```python
from build123d import *

# Parameters (mm, degrees)
SKETCH1_W                   = 57.6
SKETCH1_H                   = 31.2
BOSS_EXTRUDE1_DEPTH         = 15
FILLET1_R                   = 7.5
SHELL1_START                = -27.8
SHELL1_DEPTH                = 55.6
SKETCH4_W                   = 2.5
SKETCH4_H                   = 7.5
SKETCH4_W_2                 = 20.6
CUT_EXTRUDE1_DEPTH          = 46.03198863
SKETCH5_R                   = 1.4
CUT_EXTRUDE2_DEPTH          = 15
M3_TAPPED_HOLE1_D           = 2.5
M3_TAPPED_HOLE1_DEPTH       = 16
M3_TAPPED_HOLE1_CSINK_D     = 6
M3_TAPPED_HOLE1_CSINK_ANGLE = 90
M3_TAPPED_HOLE1_TIP         = 0.751075774


# Read off the part's stored shape, not the designer's step: Shell1
with BuildPart() as part:
    # Sketch1 → Boss-Extrude1 (new body)
    with BuildSketch(Plane(origin=(0, 0, 0), x_dir=(1, 0, 0), z_dir=(0, 1, 0))):
        Rectangle(SKETCH1_W, SKETCH1_H)
    extrude(amount=BOSS_EXTRUDE1_DEPTH)

    # Fillet1
    fillet1_edges = [part.edges().sort_by_distance(p)[0] for p in [
        (0, 15, 15.6),
        (0, 15, -15.6),
    ]]
    fillet(fillet1_edges, radius=FILLET1_R)

    # Shell1 outline → Shell1 (cut)
    with BuildSketch(Plane.YZ.offset(SHELL1_START)):
        with BuildLine():
            Line((15, -8.1), (15, 8.1))
            Line((15, 8.1), (14, 8.1))
            ThreePointArc((14, 8.1), (12.096194078, 12.696194078), (7.5, 14.6))
            Line((7.5, 14.6), (1, 14.6))
            Line((1, 14.6), (1, -14.6))
            Line((1, -14.6), (7.5, -14.6))
            ThreePointArc((7.5, -14.6), (12.096194078, -12.696194078), (14, -8.1))
            Line((14, -8.1), (15, -8.1))
        make_face()
    extrude(amount=SHELL1_DEPTH, mode=Mode.SUBTRACT)

    # Sketch4 → Cut-Extrude1 (cut, through all)
    with BuildSketch(Plane.XY.offset(15.6)):
        with Locations((-26.55, 11.25)):
            Rectangle(SKETCH4_W, SKETCH4_H)
        with Locations((0, 11.25)):
            Rectangle(SKETCH4_W_2, SKETCH4_H)
        with Locations((26.55, 11.25)):
            Rectangle(SKETCH4_W, SKETCH4_H)
    extrude(amount=-CUT_EXTRUDE1_DEPTH, mode=Mode.SUBTRACT)

    # Sketch5 → Cut-Extrude2 (cut)
    with BuildSketch(Plane(origin=(0, 1, 0), x_dir=(1, 0, 0), z_dir=(0, 1, 0))):
        with Locations(Location((0, 0, 0), (0, 0, 270))):
            Circle(SKETCH5_R)
        with Locations(Location((7.2, 0, 0), (0, 0, 270))):
            Circle(SKETCH5_R)
        with Locations(Location((-7.2, 0, 0), (0, 0, 270))):
            Circle(SKETCH5_R)
    extrude(amount=-CUT_EXTRUDE2_DEPTH, mode=Mode.SUBTRACT)

    # M3 Tapped Hole1
    with Locations(Plane(origin=(0, 1, 31.4), x_dir=(1, 0, 0), z_dir=(0, 1, 0))):
        with Locations((7.2, 31.4), (0, 31.4), (-7.2, 31.4)):
            CounterSinkHole(M3_TAPPED_HOLE1_D / 2, M3_TAPPED_HOLE1_CSINK_D / 2, depth=M3_TAPPED_HOLE1_DEPTH, counter_sink_angle=M3_TAPPED_HOLE1_CSINK_ANGLE)
            with Locations((0, 0, -(M3_TAPPED_HOLE1_DEPTH + M3_TAPPED_HOLE1_TIP / 2))):  # 118° drill point
                Cone(0, M3_TAPPED_HOLE1_D / 2, M3_TAPPED_HOLE1_TIP, mode=Mode.SUBTRACT)


solid = part.part
```
Check sheet for the modelled part. Datum: model origin and axes. Units: mm. A direction names the side the tool comes from. Give positions to 0.01 mm unless a question says otherwise; leave off trailing zeros. Order: outer loops, then holes, each group sorted by start corner. A loop starts at its lowest first (then second) coordinate and runs counter-clockwise, first axis right, second up. Notation, with made-up numbers: (44.25, -36) -> (97.25, -36) arc R31 ccw to (97.25, -7) -> close; hole circle Ø10 at (44, 30). An arc over 180 degrees is marked (long way). Return JSON: item names as keys, results as strings.
1. Material ranges on probe 1 along Z at (x, y) = (-3, 2.5); probe 2 along X at (y, z) = (9.75, 11); probe 3 along Y at (x, z) = (-14.5, -7), recorded low to high. Write a range as [from, to].
From the geometry:
{"probe 1": "[-15.6, -14.6], [14.6, 15.6]", "probe 2": "[-28.8, -27.8], [27.8, 28.8]", "probe 3": "[0, 1]"}
2. Mould release check, pull along Y, two halves, no side actions. Record for faces 4 (the cylindrical face through (-28.293, 12.745, -13.461)), 5 (the cylindrical face through (17.695, 12.045, -12.746)), 6 (the flat face through (-25.3, 12, 13)): +Y half, -Y half, draft (parallel to the pull), parting line (faces both ways), or undercut.
From the geometry:
{"face 4": "+Y half", "face 5": "undercut", "face 6": "draft"}
3. Cross-section at A-A, the plane x = -7.2. Record the cut outline in (y, z), plus the area to 3 significant figures.
From the geometry:
{"outline": "(0, -15.6) -> (7.5, -15.6) -> (7.5, -14.6) -> (1, -14.6) -> (1, -3) -> (0, -2) -> close; (0, 2) -> (1, 3) -> (1, 14.6) -> (7.5, 14.6) -> (7.5, 15.6) -> (0, 15.6) -> close", "area": "39.2 mm^2"}
4. Cross-section at D-D, the plane y = 11.75. Record the cut outline in (x, z), plus the area to 3 significant figures.
From the geometry:
{"outline": "(-28.8, -14.28) -> (-27.8, -14.28) -> (-27.8, 14.28) -> (-28.8, 14.28) -> close; (-25.3, -14.28) -> (-10.3, -14.28) -> (-10.3, -13.02) -> (-25.3, -13.02) -> close; (-25.3, 13.02) -> (-10.3, 13.02) -> (-10.3, 14.28) -> (-25.3, 14.28) -> close; (10.3, -14.28) -> (25.3, -14.28) -> (25.3, -13.02) -> (10.3, -13.02) -> close; (10.3, 13.02) -> (25.3, 13.02) -> (25.3, 14.28) -> (10.3, 14.28) -> close; (27.8, -14.28) -> (28.8, -14.28) -> (28.8, 14.28) -> (27.8, 14.28) -> close", "area": "133 mm^2"}
5. Set-up check for faces 1 (the flat face through (0, 4, -14.6)), 2 (the cylindrical face through (-17.695, 12.745, 13.461)), 3 (the flat face through (10.3, 12, -13)): record each of +Z, -Z, +X, -X, +Y, -Y from which the full face is reachable in a straight line by a thin tool's end or side.
From the geometry:
{"face 1": "none", "face 2": "+Z, +X, -X, +Y", "face 3": "+Z, -Z, +Y"}
6. Cross-section at C-C, the plane x = -24. Record the cut outline in (y, z), plus the area to 3 significant figures.
From the geometry:
{"outline": "(0, -15.6) -> (7.5, -15.6) arc R7.5 ccw to (15, -8.1) -> (14, -8.1) arc R6.5 cw to (7.5, -14.6) -> (1, -14.6) -> (1, 14.6) -> (7.5, 14.6) arc R6.5 cw to (14, 8.1) -> (15, 8.1) arc R7.5 ccw to (7.5, 15.6) -> (0, 15.6) -> close", "area": "66.2 mm^2"}
7. Go/stop test with flat-tipped pins: P1, Ø1.1, axis at x = -1.5, z = 15, coming from the +Y side; P2, Ø4, axis at x = -15, y = 13.5, coming from the +Z side; P3, Ø0.8, axis at x = 14.5, y = 14.5, coming from the -Z side. Record where each tip stops, or that it passes through.
From the geometry:
{"P1": "y = 7.5", "P2": "z = 14.44", "P3": "z = -11.66"}
8. Cross-section at B-B, the plane y = 5.75. Record the cut outline in (x, z).
From the geometry:
{"outline": "(-28.8, -15.6) -> (28.8, -15.6) -> (28.8, 15.6) -> (-28.8, 15.6) -> close; hole (-27.8, -14.6) -> (27.8, -14.6) -> (27.8, 14.6) -> (-27.8, 14.6) -> close"}
